Autodesk Fusion 360 part; units mm, degrees
sketch "Sketch1" plane through (0, 0, 0) normal (0, 0, 1) x (1, 0, 0)
  line L0 (0, 0) -> (35, 0)
  line L1 (35, 0) -> (52.5, 30.3109)
  line L2 (52.5, 30.3109) -> (35, 60.6218)
  line L3 (35, 60.6218) -> (0, 60.6218)
  line L4 (0, 60.6218) -> (-17.5, 30.3109)
  line L5 (-17.5, 30.3109) -> (0, 0)
  point P0 (17.5, 30.3109)
extrude "Extrude1" add sketch "Sketch1" along normal blind 150
shell "Shell1" thickness 2 removed faces 2 at (11.6667, 20.2073, 0) at (11.6667, 20.2073, 150)
sketch "Sketch2" plane through (0, 60.6218, 0) normal (0, 1, 0) x (-1, 0, 0)
  line L0 (-35, 0) -> (0, 0)
  line L1 (0, 0) -> (0, 150)
  line L2 (0, 150) -> (-35, 150)
  line L3 (-35, 150) -> (-35, 0)
  line L4 (-30, 144) -> (-6, 144)
  line L5 (-6, 144) -> (-6, 131)
  line L6 (-6, 131) -> (-30, 131)
  line L7 (-30, 131) -> (-30, 144)
extrude "Extrude2" cut sketch "Sketch2" against normal blind 12 contours L4 L5 L6 L7
sketch "Sketch3" plane through (0, 0, 0) normal (0, 0, 1) x (1, 0, 0)
  line L0 (0, 12) -> (0, 18)
sketch "Sketch4" plane through (26.25, -15.1554, 0) normal (0.866, -0.5, 0) x (0.5, 0.866, 0)
  line L0 (17.5, 0) -> (52.5, 0)
  line L1 (52.5, 0) -> (52.5, 150)
  line L2 (52.5, 150) -> (17.5, 150)
  line L3 (17.5, 150) -> (17.5, 0)
  line L4 (22.5, 144) -> (46.5, 144)
  line L5 (46.5, 144) -> (46.5, 131)
  line L6 (46.5, 131) -> (22.5, 131)
  line L7 (22.5, 131) -> (22.5, 144)
  point P0 (22.5, 144)
extrude "Extrude3" cut sketch "Sketch4" against normal blind 5.622 contours L4 L5 L6 L7
Can you work these out from the model? Positions are in its coordinate system, mm. A direction names the side the tool comes from. Coordinates: 2 decimals unless noted, no trailing zeros. Order: outer loops, then holes, each group sorted by start corner. A loop starts at its lowest first (then second) coordinate and runs counter-clockwise, first axis right, second up. Notation, with made-up numbers: (61.5, 28) - (107.5, 28) arc R8 cw to (107.5, 36) - close; hole circle Ø10 at (-6.75, 16). An arc over 180 degrees is marked (long way). Answer in a Markdown table with one row per item.
1. Suppose I cut it at C-C (y = 32). Please give me the cut outline in (x, z).
Reply:
| item | result |
|---|---|
| outline | (-16.52, 0) - (-14.22, 0) - (-14.22, 150) - (-16.52, 150) - close; (49.22, 0) - (51.52, 0) - (51.52, 150) - (49.22, 150) - close |
2. For faces 4 (the flat face through (42.13, 44.27, 73.95)), 5 (the flat face through (-8.628, 45.679, 73.95)), which set-ups out of +Z, -Z, +X, -X, +Y, -Y let a thin tool reach every point of the face, with its end or its side?
Reply:
| item | result |
|---|---|
| face 4 | +Z, -Z |
| face 5 | +Z, -Z, -X, +Y |
3. If we mould it in two halves opening along Y, with no side actions, what happens to faces 1 (the flat face through (43, 44, 150)), 2 (the flat face through (17, 0, 74)), 3 (the flat face through (18, 58.622, 74))? For each: pulls with the +Y half, pulls with the -Y half, needs draft (parallel to the pull), parting line crosses it, or undercut.
Reply:
| item | result |
|---|---|
| face 1 | needs draft |
| face 2 | pulls with the -Y half |
| face 3 | undercut |
4. Suppose I cut it at B-B (z = 139.5). Please give me the cut outline in (x, y).
Reply:
| item | result |
|---|---|
| outline | (-17.5, 30.31) - (0, 0) - (35, 0) - (37.5, 4.33) - (35.77, 5.33) - (33.85, 2) - (1.15, 2) - (-15.19, 30.31) - (1.15, 58.62) - (6, 58.62) - (6, 60.62) - (0, 60.62) - close; (30, 58.62) - (33.85, 58.62) - (50.19, 30.31) - (47.77, 26.11) - (49.5, 25.11) - (52.5, 30.31) - (35, 60.62) - (30, 60.62) - close |
5. Suppose I cut it at A-A (x = 10). Please give me the cut outline in (y, z), and give its area (3 significant figures).
Reply:
| item | result |
|---|---|
| outline | (0, 0) - (2, 0) - (2, 150) - (0, 150) - close; (58.62, 0) - (60.62, 0) - (60.62, 131) - (58.62, 131) - close; (58.62, 144) - (60.62, 144) - (60.62, 150) - (58.62, 150) - close |
| area | 574 mm^2 |
6. If I drill on line 1 along Y through (x, z) = (12.5, 62); line 2 along Y through (x, z) = (-9.5, 13); line 3 along X through (y, z) = (56, 109.5), over which ranges is the centre line in solid material (lowest first)?
Reply:
| item | result |
|---|---|
| line 1 | y = 0 to 2, 58.62 to 60.62 |
| line 2 | y = 16.45 to 20.45, 40.17 to 44.17 |
| line 3 | x = -2.67 to -0.36, 35.36 to 37.67 |
7. For pin 1 (4 mm diameter, centred on x = 6.5, z = 90, fed in from -Y); pin 2 (0.6 mm diameter, centred on y = 60, z = 138, fed in from +X); pin 3 (3 mm diameter, centred on y = 43.5, z = 29, fed in from +X); pin 4 (2 mm diameter, centred on y = 50, z = 94.5, fed in from -X), each with a flat end and sliding along its axis, tell me the tip position at first contact or that it passes through.
Reply:
| item | result |
|---|---|
| pin 1 | stops at y = 0 |
| pin 2 | stops at x = 35.53 |
| pin 3 | stops at x = 45.75 |
| pin 4 | stops at x = -6.71 |
8. Suppose I cut it at D-D (z = 96.5). Please give me the cut outline in (x, y).
Reply:
| item | result |
|---|---|
| outline | (-17.5, 30.31) - (0, 0) - (35, 0) - (52.5, 30.31) - (35, 60.62) - (0, 60.62) - close; hole (-15.19, 30.31) - (1.15, 2) - (33.85, 2) - (50.19, 30.31) - (33.85, 58.62) - (1.15, 58.62) - close |
